Input: part model. Units: mm. Frame: model coordinates. A direction names the side the tool comes from. Give positions to 0.01 mm unless a question says otherwise; leave off trailing zeros. Write each loop counter-clockwise with the first axis right and the second up, starting at its lowest first coordinate (ties: lowest second). Pieces come first, ordered by that corner, then holes. Notation, with made-up numbers: (26.5, 63) - (30.5, 63) arc R19 ccw to (30.5, 83) - close; hole circle Ø11 at (45.25, -13). An arc over 180 degrees is marked (long way). Answer as a JSON object with one key per item and string values. Group by question number.
from build123d import *

# Parameters (mm, degrees)
BOSS_EXTRUDE1_DEPTH   = 7.5
FILLET2_R             = 3
F_6_0MM_DOWEL_HOLE1_D = 6


with BuildPart() as part:
    # Sketch1 → Boss-Extrude1 (new, symmetric)
    with BuildSketch(Plane.XY):
        with BuildLine():
            Line((-20, 0), (-45, 0))
            Line((-45, 0), (-45, -12))
            Line((-45, -12), (-27.49545417, -12))
            ThreePointArc((-27.49545417, -12), (0, -30), (27.49545417, -12))
            Line((27.49545417, -12), (45, -12))
            Line((45, -12), (45, 0))
            Line((45, 0), (20, 0))
            ThreePointArc((20, 0), (0, -20), (-20, 0))
        make_face()
    extrude(amount=BOSS_EXTRUDE1_DEPTH, both=True)

    # Fillet2
    fillet2_edges = [part.edges().sort_by_distance(p)[0] for p in [
        (-36.247727085, -12, -7.5),
        (-45, -6, -7.5),
        (-32.5, 0, -7.5),
        (0, -20, -7.5),
        (-45, -6, 7.5),
        (-36.247727085, -12, 7.5),
        (0, -30, 7.5),
        (36.247727085, -12, 7.5),
        (45, -6, 7.5),
        (32.5, 0, 7.5),
        (0, -20, 7.5),
        (32.5, 0, -7.5),
        (-32.5, 0, 7.5),
        (45, -6, -7.5),
        (36.247727085, -12, -7.5),
        (0, -30, -7.5),
    ]]
    fillet(fillet2_edges, radius=FILLET2_R)

    # Ø6.0mm Dowel Hole1 (through all)
    with Locations(Plane(origin=(0, -12, 0), x_dir=(-1, 0, 0), z_dir=(0, -1, 0))):
        with Locations((36.247727085, 0), (-36.247727085, 0)):
            Hole(F_6_0MM_DOWEL_HOLE1_D / 2)


solid = part.part
1) Pin query (flat end, axial travel): P1, Ø8, axis at x = 11.5, z = -4.5, coming from the +Y side; P2, Ø4.5, axis at x = 35, z = 1, coming from the -Y side; P3, Ø1.5, axis at x = 5.5, y = -21, coming from the -Z side. Return the tip coordinate at first contact, or that it passes through.
2) Cut plane C-C on y = -8. Count the separate pieces of the cut face and the enclosed holes in it, and give its area (3 significant figures).
3) Cut plane B-B on x = 0. Return the cut outline in (y, z), and give its area (3 significant figures).
4) Cut plane A-A on z = 0. Return the cut outline in (x, y).
5) Mould query, pull axis X, two halves, no side actions, for faces 1 (the face through (-39.245, -5.916, -0.132)), 2 (the face through (33, 0, 0)), 3 (the face through (-45, -6, 0)). Classes: +X half, -X half, draft (parallel to the pull), parting line (faces both ways), or undercut.
6) Reachability of faces 4 (the face through (-35.09, -11.14, 6.6)), 5 (the face through (-34, -12, 3)), 6 (the face through (-35.09, -11.14, -6.6)) from +Z, -Z, +X, -X, +Y, -Y: full face, straight path, thin tool, end or side. Return the list, or none.
7) Line query: line 1 along X through (y, z) = (-3, 2.5); line 2 along Y through (x, z) = (29, -1.5); line 3 along Z through (x, y) = (8, -26). Output: solid intervals per line, ascending. Write a range as from..to.
Filled in:
{
 "1": {"P1": "stops at y = -12.64", "P2": "stops at y = -12", "P3": "stops at z = -7.45"},
 "2": {"separate pieces": "2", "enclosed holes": "2", "area": "727 mm²"},
 "3": {"outline": "(-30, -4.5) arc R3 ccw to (-27, -7.5) - (-23, -7.5) arc R3 ccw to (-20, -4.5) - (-20, 4.5) arc R3 ccw to (-23, 7.5) - (-27, 7.5) arc R3 ccw to (-30, 4.5) - close", "area": "142 mm²"},
 "4": {"outline": "(-45, -12) - (-39.25, -12) - (-39.25, 0) - (-45, 0) - close; (-33.25, -12) - (-27.5, -12) arc R30 ccw to (27.5, -12) - (33.25, -12) - (33.25, 0) - (20, 0) arc R20 cw to (-20, 0) - (-33.25, 0) - close; (39.25, -12) - (45, -12) - (45, 0) - (39.25, 0) - close"},
 "5": {"face 1": "undercut", "face 2": "draft", "face 3": "-X half"},
 "6": {"face 4": "+Z, -X, -Y", "face 5": "+Z, -Z, -X, -Y", "face 6": "-Z, -X, -Y"},
 "7": {"line 1": "x = -45..-37.91, -34.59..-19.77, 19.77..34.59, 37.91..45", "line 2": "y = -12..0", "line 3": "z = -7.49..7.49"}
}
